Here's how the part is built. I have some questions about the finished solid (model axes, mm). Face numbers are marked on the shaded views. A direction names the side the tool comes from. Coordinates: 2 decimals unless noted, no trailing zeros. Loops run counter-clockwise (first coordinate to the right, second up) from the corner with the lowest first, then second, coordinate; pieces in that order, holes last. Notation, with made-up numbers: (-17, 45.5) - (20, 45.5) arc R20 ccw to (20, 75.5) - close; hole circle Ø6 at (89.25, 2.25). An arc over 180 degrees is marked (long way). Use a Markdown table: item, result.
```python
from build123d import *

# Parameters (mm, degrees)
F0_R     = 4.306996
F0_R_2   = 6.068742
F0_R_3   = 4.632643
F0_R_4   = 4.213633
F0_R_5   = 7.585926
F1_DEPTH = 12.7


with BuildPart() as f1:
    # F0 (on Top) → F1 (new body)
    with BuildSketch(Plane.XY):
        Polygon((42.021509, 45.013756), (-47.745805, 45.013756), (-47.745805, 12.749561), (-47.745805, 5.203902), (-47.745805, -66.870145), (42.021509, -66.870145), (42.021509, 6.79579), (42.021509, 15.091317), align=None)
        with Locations((-25.889417, -15.351512)):
            Circle(F0_R, mode=Mode.SUBTRACT)
        with Locations((17.042782, -32.264195)):
            Circle(F0_R_2, mode=Mode.SUBTRACT)
        with Locations((-33.695269, 18.473854)):
            Circle(F0_R_3, mode=Mode.SUBTRACT)
        with Locations((0, 36.167122)):
            Circle(F0_R_4, mode=Mode.SUBTRACT)
        with Locations((20.945705, 24.458343)):
            Circle(F0_R_5, mode=Mode.SUBTRACT)
        Polygon((-47.745805, 5.203902), (-47.745805, 12.749561), (-70.382781, 0), (-74.806102, 3.382537), (-77.392745, 0), (-73.244929, -6.244683), (-77.091641, -8.799729), (-74.813173, -12.230043), (-66.479854, -9.10683), (-67.997565, -5.057293), align=None)
        Polygon((66.740051, 4.423317), (42.021509, 15.091317), (42.021509, 6.79579), (66.344172, -2.770602), (69.478922, -11.232767), (76.180932, -8.750055), (73.244929, -6.504878), (76.627463, -2.081561), (80.270201, 0), (80.270201, 4.423317), align=None)
    extrude(amount=F1_DEPTH)


solid = f1.part
```
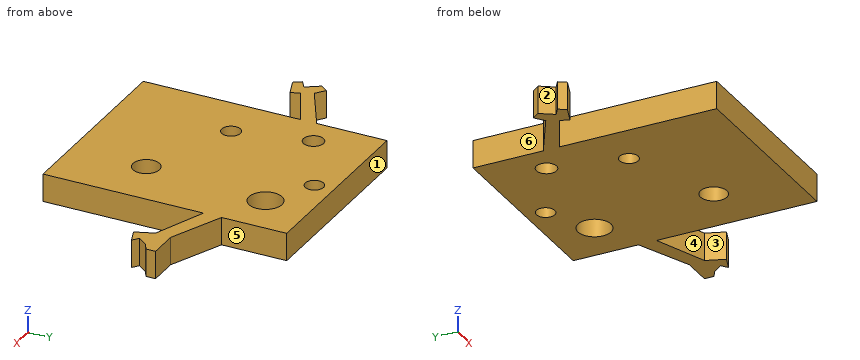
Q1. I want a section at B-B, the plane y = -34. Write out the boundary of the cut face in (x, z), then the cut area to 3 significant figures.
Check values:
| item | result |
|---|---|
| outline | (-47.75, 0) - (11.23, 0) - (11.23, 12.7) - (-47.75, 12.7) - close; (22.86, 0) - (42.02, 0) - (42.02, 12.7) - (22.86, 12.7) - close |
| area | 992 mm^2 |
Q2. I want a section at A-A, the plane x = 0. Write out the boundary of the cut face in (y, z), then the cut area to 3 significant figures.
Check values:
| item | result |
|---|---|
| outline | (-66.87, 0) - (31.95, 0) - (31.95, 12.7) - (-66.87, 12.7) - close; (40.38, 0) - (45.01, 0) - (45.01, 12.7) - (40.38, 12.7) - close |
| area | 1,310 mm^2 |
Q3. If we mould it in two halves opening along Y, with no side actions, what happens to the marked faces 1, 2 and 3? For each: pulls with the +Y half, pulls with the -Y half, needs draft (parallel to the pull), parting line crosses it, or undercut.
Check values:
| item | result |
|---|---|
| face 1 | pulls with the +Y half |
| face 2 | undercut |
| face 3 | pulls with the -Y half |
Q4. Which directions (+Z, -Z, +X, -X, +Y, -Y) give clear straight access to the entire face, cutting with the end or side of a thin tool? Please do the marked faces 4, 5 and 6.
Check values:
| item | result |
|---|---|
| face 4 | +Z, -Z, -Y |
| face 5 | +Z, -Z, +X, +Y |
| face 6 | +Z, -Z, -X, +Y |
Q5. Will these pins go through, and if not, where does the flat tip stop? P1, Ø4, axis at y = 29, z = 9, coming from the -X side; P2, Ø4, axis at x = 60, z = 8.5, coming from the +Y side; P3, Ø9, axis at x = 20.95, y = 24.46, coming from the +Z side; P4, Ø6, axis at y = -37, z = 9, coming from the +X side.
Check values:
| item | result |
|---|---|
| P1 | x = -47.75 |
| P2 | y = 8.2 |
| P3 | through |
| P4 | x = 42.02 |
Q6. I want a section at D-D, the plane y = 21.5. Write out the boundary of the cut face in (x, z).
Check values:
| item | result |
|---|---|
| outline | (-47.75, 0) - (-37.2, 0) - (-37.2, 12.7) - (-47.75, 12.7) - close; (-30.19, 0) - (13.96, 0) - (13.96, 12.7) - (-30.19, 12.7) - close; (27.93, 0) - (42.02, 0) - (42.02, 12.7) - (27.93, 12.7) - close |
Q7. Please list where these lines run through material, in increasing order: L1, parallel to X at y = 17.5, z = 9.75; L2, parallel to X at y = -3, z = 11.5; L3, parallel to X at y = -32, z = 0.75. Write a range as from..to.
Check values:
| item | result |
|---|---|
| L1 | -47.75..-38.22, -29.17..17.92, 23.97..42.02 |
| L2 | -75.4..-63.94, -47.75..42.02, 66.43..75.93 |
| L3 | -47.75..10.98, 23.11..42.02 |
Q8. I want a section at C-C, the plane z = 10. Give the number of separate pieces and of enclosed holes in the cut face, then the cut area to 3 significant figures.
Check values:
| item | result |
|---|---|
| separate pieces | 1 |
| enclosed holes | 5 |
| area | 10,100 mm^2 |
